```python
from build123d import *

# Parameters (mm, degrees)
EXTRUDE_2_DEPTH     = 5
SKETCH_5_R          = 40
EXTRUDE_5_DEPTH     = 100
EXTRUDE_6_DEPTH     = 100
CUT_EXTRUDE_1_DEPTH = 10
CUT_EXTRUDE_2_DEPTH = 10
CUT_EXTRUDE_3_DEPTH = 10
CUT_EXTRUDE_4_DEPTH = 10
SKETCH_11_R         = 40
EXTRUDE_7_DEPTH     = 690
SKETCH_12_R         = 90
EXTRUDE_8_DEPTH     = 10
SKETCH_13_R         = 40
EXTRUDE_9_DEPTH     = 100


with BuildPart() as part:
    # 草图1 → 凸台-拉伸2 (new body)
    with BuildSketch(Plane(origin=(0, 0, 0), x_dir=(1, 0, 0), z_dir=(0, 1, 0))):
        with BuildLine():
            Line((100, -125), (-100, -125))
            Line((-100, -125), (-100, 125))
            Line((-100, 125), (100, 125))
            ThreePointArc((100, 125), (225, 0), (100, -125))
        make_face()
    extrude(amount=EXTRUDE_2_DEPTH)

    # 草图5 → 凸台-拉伸5 (add)
    with BuildSketch(Plane(origin=(0, 5, 0), x_dir=(1, 0, 0), z_dir=(0, 1, 0))):
        with Locations((100, 0)):
            Circle(SKETCH_5_R)
    extrude(amount=EXTRUDE_5_DEPTH)

    # 草图6 → 凸台-拉伸6 (add)
    with BuildSketch(Plane(origin=(0, 5, 0), x_dir=(1, 0, 0), z_dir=(0, 1, 0))):
        with BuildLine():
            Line((102.5, -100), (97.5, -100))
            Line((97.5, -100), (97.5, -39.921798557))
            ThreePointArc((97.5, -39.921798557), (100, -40), (102.5, -39.921798557))
            Line((102.5, -39.921798557), (102.5, -100))
        make_face()
        with BuildLine():
            Line((0, -2.5), (0, 2.5))
            Line((0, 2.5), (60.078201443, 2.5))
            ThreePointArc((60.078201443, 2.5), (60, 0), (60.078201443, -2.5))
            Line((60.078201443, -2.5), (0, -2.5))
        make_face()
        with BuildLine():
            Line((102.5, 100), (97.5, 100))
            Line((97.5, 100), (97.5, 39.921798557))
            ThreePointArc((97.5, 39.921798557), (100, 40), (102.5, 39.921798557))
            Line((102.5, 39.921798557), (102.5, 100))
        make_face()
        with BuildLine():
            Line((200, -2.5), (200, 2.5))
            Line((200, 2.5), (139.921798557, 2.5))
            ThreePointArc((139.921798557, 2.5), (140, 0), (139.921798557, -2.5))
            Line((139.921798557, -2.5), (200, -2.5))
        make_face()
    extrude(amount=EXTRUDE_6_DEPTH)

    # 草图7 → 切除-拉伸1 (cut)
    with BuildSketch(Plane.ZY.offset(-97.5)):
        Polygon((39.921798557, 105), (100, 5), (100, 105), align=None)
    extrude(amount=-CUT_EXTRUDE_1_DEPTH, mode=Mode.SUBTRACT)

    # 草图8 → 切除-拉伸2 (cut)
    with BuildSketch(Plane.XY.offset(2.5)):
        Polygon((139.921798557, 105), (200, 5), (200, 105), align=None)
    extrude(amount=-CUT_EXTRUDE_2_DEPTH, mode=Mode.SUBTRACT)

    # 草图9 → 切除-拉伸3 (cut)
    with BuildSketch(Plane(origin=(102.5, 0, 0), x_dir=(0, 0, -1), z_dir=(1, 0, 0))):
        Polygon((39.921798557, 105), (100, 105), (100, 5), align=None)
    extrude(amount=-CUT_EXTRUDE_3_DEPTH, mode=Mode.SUBTRACT)

    # 草图10 → 切除-拉伸4 (cut)
    with BuildSketch(Plane(origin=(0, 0, -2.5), x_dir=(-1, 0, 0), z_dir=(0, 0, -1))):
        Polygon((0, 105), (0, 5), (-60.078201443, 105), align=None)
    extrude(amount=-CUT_EXTRUDE_4_DEPTH, mode=Mode.SUBTRACT)

    # 草图11 → 凸台-拉伸7 (add)
    with BuildSketch(Plane(origin=(0, 105, 0), x_dir=(1, 0, 0), z_dir=(0, 1, 0))):
        with Locations((100, 0)):
            Circle(SKETCH_11_R)
    extrude(amount=EXTRUDE_7_DEPTH)

    # 草图12 → 凸台-拉伸8 (add)
    with BuildSketch(Plane(origin=(0, 795, 0), x_dir=(1, 0, 0), z_dir=(0, 1, 0))):
        with Locations((100, 0)):
            Circle(SKETCH_12_R)
    extrude(amount=EXTRUDE_8_DEPTH)

    # 草图13 → 凸台-拉伸9 (add)
    with BuildSketch(Plane(origin=(0, 805, 0), x_dir=(1, 0, 0), z_dir=(0, 1, 0))):
        with Locations((100, 0)):
            Circle(SKETCH_13_R)
    extrude(amount=EXTRUDE_9_DEPTH)


solid = part.part
```
Geometry: final body of the model. Coordinates: model frame, mm. A direction names the side the tool comes from. Round coordinates to 2 decimals unless told otherwise and drop trailing zeros. Loops run counter-clockwise (first coordinate to the right, second up) from the corner with the lowest first, then second, coordinate; pieces in that order, holes last.
Item 1: Section D-D, the plane y = 620. Output: boundary loops of the cut face in (x, z), plus the area to 3 significant figures.
Checked values:
outline: circle Ø80 at (100, 0)
area: 5,030 mm2
Item 2: Line query: L1, parallel to Y at x = 156, z = 4; L2, parallel to Y at x = 193, z = 19; L3, parallel to Z at x = 79.5, y = 728.5. Output: solid intervals per line, ascending.
Checked values:
L1: y = 0 to 5, 795 to 805
L2: y = 0 to 5
L3: z = -34.35 to 34.35
Item 3: Reachability of faces 1 (the flat face through (100.04, 54.3, -70.38)), 2 (the flat face through (102.5, 43, -63)), 3 (the flat face through (29, 5, -30)), 4 (the flat face through (169.54, 55.7, 0.04)), 5 (the flat face through (29.62, 54.3, -0.04)) from +Z, -Z, +X, -X, +Y, -Y: full face, straight path, thin tool, end or side. Return the list, or none.
Checked values:
face 1: -Z, +X, -X
face 2: -Z, +X
face 3: none
face 4: +Z, -Z, +X
face 5: +Z, -Z, -X
Item 4: Section A-A, the plane z = -62. Output: boundary loops of the cut face in (x, y), plus the area to 3 significant figures.
Checked values:
outline: (-100, 0) - (208.54, 0) - (208.54, 5) - (102.5, 5) - (102.5, 68.25) - (97.5, 68.25) - (97.5, 5) - (-100, 5) - close; (34.76, 795) - (165.24, 795) - (165.24, 805) - (34.76, 805) - close
area: 3,160 mm2
Item 5: Mould query, pull axis Y, two halves, no side actions, for faces 6 (the flat face through (99, 905, -1)), 7 (the flat face through (99.96, 55.7, 69.54)), 8 (the cylindrical face through (138.153, 854.3, -12.015)), 9 (the flat face through (97.5, 32, -57)). Classes: released by +Y, released by -Y, zero draft, split by the parting line, or undercut.
Checked values:
face 6: released by +Y
face 7: undercut
face 8: zero draft
face 9: undercut
Item 6: Section B-B, the plane x = -51.5. Output: boundary loops of the cut face in (y, z), plus the area to 3 significant figures.
Checked values:
outline: (0, -125) - (5, -125) - (5, 125) - (0, 125) - close
area: 1,250 mm2
Item 7: Contact query for flat-ended pins moving along their axis: P1, Ø3, axis at y = 631.5, z = -9.5, coming from the +X side; P2, Ø1.5, axis at y = 580, z = 19.5, coming from the -X side; P3, Ø18, axis at x = 31, y = 73.5, coming from the -Z side; P4, Ø6, axis at x = 114.5, z = -53, coming from the -Y side. Output: stop coordinate, or through.
Checked values:
P1: stops at x = 139.19
P2: stops at x = 64.67
P3: stops at z = -2.5
P4: stops at y = 0
Item 8: Section C-C, the plane z = 61.5. Output: boundary loops of the cut face in (x, y), plus the area to 3 significant figures.
Checked values:
outline: (-100, 0) - (208.82, 0) - (208.82, 5) - (102.5, 5) - (102.5, 69.08) - (97.5, 69.08) - (97.5, 5) - (-100, 5) - close; (34.29, 795) - (165.71, 795) - (165.71, 805) - (34.29, 805) - close
area: 3,180 mm2
